```python
from build123d import *

# Parameters (mm, degrees)
SKETCH_W        = 6.5
SKETCH_H        = 6.5
PAD_DEPTH       = 1.05
SKETCH001_W     = 1.75
SKETCH001_H     = 1.75
PAD001_DEPTH    = 0.5
SKETCH002_W     = 1
SKETCH002_H     = 1
PAD002_DEPTH    = 2.7
SKETCH003_R     = 0.5
PAD003_DEPTH    = 3.2
CHAMFER_SIZE    = 0.08
SKETCH004_R     = 3.05
PAD004_DEPTH    = 1.5
SKETCH005_W     = 6.5
SKETCH005_H     = 6.5
PAD005_DEPTH    = 6.5
SKETCH006_R     = 2.675
PAD006_DEPTH    = 5.6
SKETCH007_R     = 3.125
PAD007_DEPTH    = 3.7
SKETCH008_R     = 2.675
PAD008_DEPTH    = 0.8
CHAMFER001_SIZE = 0.08
CHAMFER002_SIZE = 0.2
SKETCH009_R     = 2.3
POCKET_DEPTH    = 2
SKETCH010_R     = 0.25
POCKET001_DEPTH = 3


with BuildPart() as part:
    # Sketch → Pad (new body)
    with BuildSketch(Plane.XY.offset(0.5)):
        Rectangle(SKETCH_W, SKETCH_H)
    extrude(amount=PAD_DEPTH)

    # Sketch001 (on Face5 of Pad) → Pad001 (join)
    with BuildSketch(Plane(origin=(0, 0, 0.5), x_dir=(1, 0, 0), z_dir=(0, 0, -1))):
        with Locations((-2.375, 2.375)):
            Rectangle(SKETCH001_W, SKETCH001_H)
        with Locations((-2.375, -2.375)):
            Rectangle(SKETCH001_W, SKETCH001_H)
        with Locations((2.375, -2.375)):
            Rectangle(SKETCH001_W, SKETCH001_H)
        with Locations((2.375, 2.375)):
            Rectangle(SKETCH001_W, SKETCH001_H)
    extrude(amount=PAD001_DEPTH)

    # Sketch002 (on Face26 of Pad001) → Pad002 (join)
    with BuildSketch(Plane(origin=(0, 0, 0), x_dir=(1, 0, 0), z_dir=(0, 0, -1))):
        with Locations((-2.54, 2.54)):
            Rectangle(SKETCH002_W, SKETCH002_H)
        with Locations((2.54, 2.54)):
            Rectangle(SKETCH002_W, SKETCH002_H)
        with Locations((2.54, -2.54)):
            Rectangle(SKETCH002_W, SKETCH002_H)
        with Locations((-2.54, -2.54)):
            Rectangle(SKETCH002_W, SKETCH002_H)
    extrude(amount=PAD002_DEPTH)

    # Sketch003 (on Face5 of Pad002) → Pad003 (join)
    with BuildSketch(Plane(origin=(0, 0, 0.5), x_dir=(1, 0, 0), z_dir=(0, 0, -1))):
        Circle(SKETCH003_R)
    extrude(amount=PAD003_DEPTH)

    # Chamfer
    chamfer_edges = [part.edges().sort_by_distance(p)[0] for p in [
        (-0.5, 0, -2.7),
    ]]
    chamfer(chamfer_edges, length=CHAMFER_SIZE)

    # Sketch004 (on Face20 of Chamfer) → Pad004 (join)
    with BuildSketch(Plane.XY.offset(1.55)):
        Circle(SKETCH004_R)
    extrude(amount=PAD004_DEPTH)

    # Sketch005 (on Face48 of Pad004) → Pad005 (join)
    with BuildSketch(Plane.XY.offset(3.05)):
        Rectangle(SKETCH005_W, SKETCH005_H)
    extrude(amount=PAD005_DEPTH)

    # Sketch006 (on Face2 of Pad005) → Pad006 (join)
    with BuildSketch(Plane(origin=(-3.25, 0, 0), x_dir=(0, -1, 0), z_dir=(-1, 0, 0))):
        with Locations((0, 6.3)):
            Circle(SKETCH006_R)
    extrude(amount=PAD006_DEPTH)

    # Sketch007 (on Face9 of Pad006) → Pad007 (join)
    with BuildSketch(Plane(origin=(-8.85, 0, 0), x_dir=(0, -1, 0), z_dir=(-1, 0, 0))):
        with Locations((0, 6.3)):
            Circle(SKETCH007_R)
    extrude(amount=PAD007_DEPTH)

    # Sketch008 (on Face3 of Pad007) → Pad008 (join)
    with BuildSketch(Plane(origin=(-12.55, 0, 0), x_dir=(0, -1, 0), z_dir=(-1, 0, 0))):
        with Locations((0, 6.3)):
            Circle(SKETCH008_R)
    extrude(amount=PAD008_DEPTH)

    # Chamfer001
    chamfer001_edges = [part.edges().sort_by_distance(p)[0] for p in [
        (-13.35, 2.675, 6.3),
    ]]
    chamfer(chamfer001_edges, length=CHAMFER001_SIZE)

    # Chamfer002
    chamfer002_edges = [part.edges().sort_by_distance(p)[0] for p in [
        (-8.85, 3.125, 6.3),
        (-12.55, 3.125, 6.3),
    ]]
    chamfer(chamfer002_edges, length=CHAMFER002_SIZE)

    # Sketch009 (on Face7 of Chamfer002) → Pocket (cut)
    with BuildSketch(Plane(origin=(-13.35, 0, 0), x_dir=(0, -1, 0), z_dir=(-1, 0, 0))):
        with Locations((0, 6.3)):
            Circle(SKETCH009_R)
    extrude(amount=-POCKET_DEPTH, mode=Mode.SUBTRACT)

    # Sketch010 (on Face11 of Pocket) → Pocket001 (cut)
    with BuildSketch(Plane(origin=(-11.35, 0, 0), x_dir=(0, -1, 0), z_dir=(-1, 0, 0))):
        with Locations((0, 6.3)):
            Circle(SKETCH010_R)
    extrude(amount=-POCKET001_DEPTH, mode=Mode.SUBTRACT)

    # Sketch011 → Groove (revolve, cut)
    with BuildSketch(Plane.XZ):
        with BuildLine():
            ThreePointArc((0, 10.289421), (-2.380676, 9.806619), (-4.681284, 9.026929))
            Line((-4.681284, 9.026929), (-4.681284, 13.840189))
            Line((-4.681284, 13.840189), (0, 13.840189))
            Line((0, 13.840189), (0, 10.289421))
        make_face()
    revolve(axis=Axis((0, 0, 0), (0, 0, 1)), mode=Mode.SUBTRACT)


solid = part.part
```
Input: part model. Units: mm. Frame: model coordinates. A direction names the side the tool comes from. Give positions to 0.01 mm unless a question says otherwise; leave off trailing zeros. Loops run counter-clockwise (first coordinate to the right, second up) from the corner with the lowest first, then second, coordinate; pieces in that order, holes last. Notation, with made-up numbers: (43, 60) -> (56, 60) arc R31 cw to (56, 92) -> close; hole circle Ø9 at (58, 2). An arc over 180 degrees is marked (long way). Use a Markdown table: item, result.
Q1. First-contact query: P1, Ø1.1, axis at y = 2.5, z = -1, coming from the -X side; P2, Ø1.1, axis at y = 2.5, z = -0.5, coming from the -X side; P3, Ø1.1, axis at x = -2.5, z = -2, coming from the +Y side. Flat tips, straight axial feed; report the tip coordinate or a pass-through.
Entries:
| item | result |
|---|---|
| P1 | stops at x = -3.04 |
| P2 | stops at x = -3.25 |
| P3 | stops at y = 3.04 |
Q2. Section query C-C, the plane x = -10.5. Return the cut outline in (y, z) (3 decimals), plus the area to 3 significant figures.
Entries:
| item | result |
|---|---|
| outline | circle Ø6.25 at (0, 6.3); hole circle Ø0.5 at (0, 6.3) |
| area | 30.5 mm² |
Q3. Pull-direction query (Y, two-part tool) for faces 5 (the flat face through (-2.5, -2.04, -1.3)), 6 (the flat face through (0, -3.25, 1)), 7 (the flat face through (2.5, -2.5, -2.7)); classes: pulls with the +Y half, pulls with the -Y half, needs draft (parallel to the pull), parting line crosses it, or undercut.
Entries:
| item | result |
|---|---|
| face 5 | undercut |
| face 6 | pulls with the -Y half |
| face 7 | needs draft |
Q4. Ray query, probe 1 along Z at (x, y) = (-12.1, 0) (3 decimals); probe 2 along Z at (x, y) = (-12.75, 0) (3 decimals); probe 3 along X at (y, z) = (-1, 6). Return the intervals inside material, ascending. Write a range as from..to.
Entries:
| item | result |
|---|---|
| probe 1 | z = 3.175..4, 8.6..9.425 |
| probe 2 | z = 3.625..4, 8.6..8.975 |
| probe 3 | x = -11.35..3.25 |
Q5. Section query A-A, the plane z = -0.5. Return the cut outline in (x, y).
Entries:
| item | result |
|---|---|
| outline | (-3.04, -3.04) -> (-2.04, -3.04) -> (-2.04, -2.04) -> (-3.04, -2.04) -> close; (-3.04, 2.04) -> (-2.04, 2.04) -> (-2.04, 3.04) -> (-3.04, 3.04) -> close; circle Ø1 at (0, 0); (2.04, -3.04) -> (3.04, -3.04) -> (3.04, -2.04) -> (2.04, -2.04) -> close; (2.04, 2.04) -> (3.04, 2.04) -> (3.04, 3.04) -> (2.04, 3.04) -> close |
Q6. Section query D-D, the plane x = -6.5. Return the cut outline in (y, z) (3 decimals).
Entries:
| item | result |
|---|---|
| outline | circle Ø5.35 at (0, 6.3) |
Q7. Access query for faces 1 (the flat face through (-3.25, -0.05, 9.14)), 2 (the flat face through (2.04, 2.5, -1.3)), 3 (the flat face through (-3.04, 2.5, -1.3)), 4 (the flat face through (3.04, -2.5, -1.3)). Directions: +Z, -Z, +X, -X, +Y, -Y. A direction counts if a zero-diameter tool reaches every point of the face in a straight line with its end or side. Return the directions, or none.
Entries:
| item | result |
|---|---|
| face 1 | none |
| face 2 | -Z, +Y, -Y |
| face 3 | -Z, -X, +Y, -Y |
| face 4 | -Z, +X, +Y, -Y |
